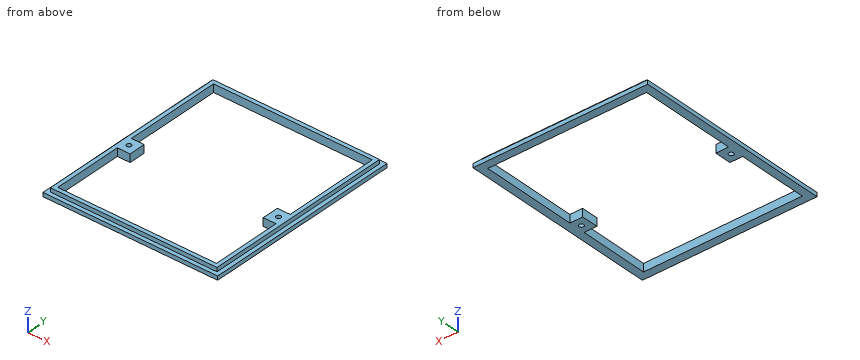
```python
from build123d import *

# Parameters (mm, degrees)
SKETCH_W             = 105
SKETCH_H             = 120
PAD_DEPTH            = 2.4
POCKET001_DEPTH      = 2.401
POCKET001_DEPTH_BACK = -0.001
SKETCH026_W          = 100.2
SKETCH026_H          = 115.2
PAD001_DEPTH         = 2.4
SKETCH024_R          = 1.4
POCKET_DEPTH         = 5


with BuildPart() as part:
    # Sketch → Pad (new body)
    with BuildSketch(Plane.XY):
        with Locations((0, -10)):
            Rectangle(SKETCH_W, SKETCH_H)
    extrude(amount=PAD_DEPTH)

    # Sketch025 → Pocket001 (cut, two sides)
    with BuildSketch(Plane.XY.offset(2.4)) as pocket001_sk:
        Polygon((-47.7, 45.2), (-47.7, -13), (-40, -13), (-40, -23), (-47.7, -23), (-47.7, -65.2), (47.7, -65.2), (47.7, -23), (40, -23), (40, -13), (47.7, -13), (47.7, 45.2), align=None)
    extrude(amount=-POCKET001_DEPTH, mode=Mode.SUBTRACT)
    extrude(pocket001_sk.sketch, amount=-POCKET001_DEPTH_BACK, mode=Mode.SUBTRACT)

    # Sketch026 → Pad001 (new body)
    with BuildSketch(Plane.XY.offset(2.4)):
        with Locations((0, -10)):
            Rectangle(SKETCH026_W, SKETCH026_H)
        Polygon((-47.7, 45.2), (-47.7, -13), (-40, -13), (-40, -23), (-47.7, -23), (-47.7, -65.2), (47.7, -65.2), (47.7, -23), (40, -23), (40, -13), (47.7, -13), (47.7, 45.2), align=None, mode=Mode.SUBTRACT)
    extrude(amount=PAD001_DEPTH)

    # Sketch024 → Pocket (cut)
    with BuildSketch(Plane.XY.offset(4.8)):
        with Locations((-45, -18)):
            Circle(SKETCH024_R)
        with Locations((45, -18)):
            Circle(SKETCH024_R)
    extrude(amount=-POCKET_DEPTH, mode=Mode.SUBTRACT)


solid = part.part
```
Could you check a few things on this model? Use its own coordinates, in mm. Round coordinates to 2 decimals unless told otherwise and drop trailing zeros. Loops run counter-clockwise (first coordinate to the right, second up) from the corner with the lowest first, then second, coordinate; pieces in that order, holes last. Notation, with made-up numbers: (7, 71) - (46, 71) arc R36 cw to (46, 110) - close; hole circle Ø2 at (26.25, 71.5). An arc over 180 degrees is marked (long way). Answer in a Markdown table with one row per item. Add a question column.
(1) If we section it at D-D (y = 34): Please give me the cut outline in (x, z).
(2) I'm going to push flat-ended pins straight in: pin 1 (1.2 mm diameter, centred on x = -18.5, z = 3.5, fed in from +Y); pin 2 (1.4 mm diameter, centred on y = -41, z = 3.5, fed in from -X); pin 3 (0.7 mm diameter, centred on y = -24.5, z = 3.5, fed in from +X). Where does each tip first touch, or does it pass through?
(3) I need wall thicknesses on line 1 along Y through (x, z) = (-45, 3.5); line 2 along Y through (x, z) = (-3, 2.3); line 3 along X through (y, z) = (21.5, 2.75). Which ranges of each line are inside material? Lowest first, please.
(4) If we section it at B-B (y = -18): Please give me the cut outline in (x, z), plus the area to 3 significant figures.
(5) If we section it at A-A (x = -31.5): Please give me the cut outline in (y, z), plus the area to 3 significant figures.
(6) If we section it at C-C (x = 45): Please give me the cut outline in (y, z).
Model answer:
| question | item | result |
|---|---|---|
| 1 | outline | (-52.5, 0) - (-47.7, 0) - (-47.7, 4.8) - (-50.1, 4.8) - (-50.1, 2.4) - (-52.5, 2.4) - close; (47.7, 0) - (52.5, 0) - (52.5, 2.4) - (50.1, 2.4) - (50.1, 4.8) - (47.7, 4.8) - close |
| 2 | pin 1 | stops at y = 47.6 |
| 2 | pin 2 | stops at x = -50.1 |
| 2 | pin 3 | stops at x = 50.1 |
| 3 | line 1 | y = -67.6 to -65.2, -23 to -19.4, -16.6 to -13, 45.2 to 47.6 |
| 3 | line 2 | y = -70 to -65.2, 45.2 to 50 |
| 3 | line 3 | x = -50.1 to -47.7, 47.7 to 50.1 |
| 4 | outline | (-52.5, 0) - (-46.4, 0) - (-46.4, 4.8) - (-50.1, 4.8) - (-50.1, 2.4) - (-52.5, 2.4) - close; (-43.6, 0) - (-40, 0) - (-40, 4.8) - (-43.6, 4.8) - close; (40, 0) - (43.6, 0) - (43.6, 4.8) - (40, 4.8) - close; (46.4, 0) - (52.5, 0) - (52.5, 2.4) - (50.1, 2.4) - (50.1, 4.8) - (46.4, 4.8) - close |
| 4 | area | 81.6 mm² |
| 5 | outline | (-70, 0) - (-65.2, 0) - (-65.2, 4.8) - (-67.6, 4.8) - (-67.6, 2.4) - (-70, 2.4) - close; (45.2, 0) - (50, 0) - (50, 2.4) - (47.6, 2.4) - (47.6, 4.8) - (45.2, 4.8) - close |
| 5 | area | 34.6 mm² |
| 6 | outline | (-70, 0) - (-65.2, 0) - (-65.2, 4.8) - (-67.6, 4.8) - (-67.6, 2.4) - (-70, 2.4) - close; (-23, 0) - (-19.4, 0) - (-19.4, 4.8) - (-23, 4.8) - close; (-16.6, 0) - (-13, 0) - (-13, 4.8) - (-16.6, 4.8) - close; (45.2, 0) - (50, 0) - (50, 2.4) - (47.6, 2.4) - (47.6, 4.8) - (45.2, 4.8) - close |
